Here's how the part is built. I have some questions about the finished solid (model axes, mm). A direction names the side the tool comes from. Coordinates: 2 decimals unless noted, no trailing zeros. Write each loop counter-clockwise with the first axis right and the second up, starting at its lowest first coordinate (ties: lowest second). Pieces come first, ordered by that corner, then holes. Notation, with made-up numbers: (-2.75, 1) -> (30.25, 1) arc R28 ccw to (30.25, 36) -> close; hole circle Ø1 at (1, -35). An arc over 180 degrees is marked (long way). Use a Markdown table: item, result. Add a question column.
Item 1: If I drill on line 1 along Z through (x, y) = (8.25, 7.5) (3 decimals); line 2 along X through (y, z) = (6.4, 6); line 3 along Z through (x, y) = (-1.75, 7), over which ranges is the centre line in solid material (lowest first)? Write a range as from..to.
Item 2: Imagine slicing it at D-D, the plane y = 9.5. Write out the boundary of the cut face in (x, z), and give its area (3 significant figures).
Item 3: Imagine slicing it at B-B, the plane y = 7.5. Write out the boundary of the cut face in (x, z) (3 decimals).
Item 4: On a 3-axis mill with a long thin cutter (end or side, diameter ignored), from which of +Z, -Z, +X, -X, +Y, -Y can I reach the whole of each face in a straight line? I mean faces 4 (the flat face through (-1.7, 9.5, 11.5)), 5 (the flat face through (-2, 10, 4)), 6 (the flat face through (-1.8, 5.5, 11.5)). Say none if no direction works.
Item 5: If we mould it in two halves opening along Y, with no side actions, what happens to faces 1 (the cylindrical face through (9.43, 6.63, 6.11)), 2 (the flat face through (-2, 5, 4)), 3 (the flat face through (8, 8, 0))? For each: pulls with the +Y half, pulls with the -Y half, needs draft (parallel to the pull), parting line crosses it, or undercut.
Item 6: Imagine slicing it at C-C, the plane x = -1.75. Write out the boundary of the cut face in (y, z), and give its area (3 significant figures).
Item 7: Imagine slicing it at A-A, the plane z = 6. Write out the boundary of the cut face in (x, y) (3 decimals).
Item 8: Will these pins go through, and if not, where does the flat tip stop? pin 1 Ø1.8 at (x, z) = (-2, 3) entering from -Y; pin 2 Ø6.5 at (y, z) = (13.5, 4) entering from -X; pin 3 Ø1.8 at (x, z) = (-1.5, 4.5) entering from +Y.
Autodesk Fusion 360 part; units mm, degrees
sketch "Sketch1" plane through (0, 0, 0) normal (0, 0, 1) x (1, 0, 0)
  line L0 (0, 0) -> (20, 0)
  line L1 (20, 0) -> (20, 15)
  line L2 (20, 15) -> (0, 15)
  line L3 (0, 15) -> (0, 0)
  dimension "d1" = 15
sketch "Sketch2" plane through (0, 0, 0) normal (0, 0, 1) x (1, 0, 0)
  line L0 (0, 10) -> (-3.5, 10)
  line L1 (-3.5, 10) -> (-3.5, 5)
  line L2 (-3.5, 5) -> (0, 5)
  line L3 (0, 5) -> (0, 10)
  dimension "d2" = 3.5
extrude "Extrude1" add sketch "Sketch1" sketch "Sketch2" along normal blind 12 of sketch 2
chamfer "Chamfer1" distance 3 angle 45 1 edges at (10, 0, 12)
chamfer "Chamfer2" distance 3 angle 45 1 edges at (10, 15, 12)
hole "Hole1" at (-1.75, 5, 6) direction (0, 1, 0) diameter 2.5 depth 9 tip angle 118
hole "Hole2" at (20, 7.5, 6) direction (-1, 0, 0) diameter 1.75 depth 38 tip angle 118
chamfer "Chamfer3" distance 3 angle 45 1 edges at (20, 7.5, 12)
chamfer "Chamfer4" distance 1 angle 45 2 edges at (-1.75, 5, 12) (-1.75, 10, 12)
Ans:
| question | item | result |
|---|---|---|
| 1 | line 1 | z = 0..5.125, 6.875..12 |
| 1 | line 2 | x = -3.5..-3, -0.5..20 |
| 1 | line 3 | z = 0..4.75, 7.25..12 |
| 2 | outline | (-3.5, 0) -> (20, 0) -> (20, 9) -> (17, 12) -> (0, 12) -> (0, 11.5) -> (-3.5, 11.5) -> close; hole circle Ø2.5 at (-1.75, 6) |
| 2 | area | 271 mm^2 |
| 3 | outline | (-3.5, 0) -> (20, 0) -> (20, 5.125) -> (-0.857, 5.125) arc R1.25 cw to (-2.643, 5.125) -> (-3.5, 5.125) -> close; (-3.5, 6.875) -> (-2.643, 6.875) arc R1.25 cw to (-0.857, 6.875) -> (20, 6.875) -> (20, 9) -> (17, 12) -> (-3.5, 12) -> close |
| 4 | face 4 | +Z, -X, +Y |
| 4 | face 5 | +Z, -Z, -X, +Y |
| 4 | face 6 | +Z, -X, -Y |
| 5 | face 1 | undercut |
| 5 | face 2 | pulls with the -Y half |
| 5 | face 3 | needs draft |
| 6 | outline | (5, 0) -> (10, 0) -> (10, 4.75) -> (5, 4.75) -> close; (5, 7.25) -> (10, 7.25) -> (10, 11) -> (9, 12) -> (6, 12) -> (5, 11) -> close |
| 6 | area | 46.5 mm^2 |
| 7 | outline | (-3.5, 5) -> (-3, 5) -> (-3, 6.625) -> (-3.5, 6.625) -> close; (-3.5, 8.375) -> (-3, 8.375) -> (-3, 10) -> (-3.5, 10) -> close; (-0.5, 5) -> (0, 5) -> (0, 0) -> (20, 0) -> (20, 6.625) -> (-0.5, 6.625) -> close; (-0.5, 8.375) -> (20, 8.375) -> (20, 15) -> (0, 15) -> (0, 10) -> (-0.5, 10) -> close |
| 8 | pin 1 | stops at y = 5 |
| 8 | pin 2 | stops at x = 0 |
| 8 | pin 3 | stops at y = 10 |
